Autodesk Inventor part; units mm, degrees
ref_plane "YZ Plane" through (0, 0, 0) normal (1, 0, 0) x (0, 1, 0)
ref_plane "XZ Plane" through (0, 0, 0) normal (0, 1, 0) x (-1, 0, 0)
ref_plane "XY Plane" through (0, 0, 0) normal (0, 0, 1) x (1, 0, 0)
sketch "Sketch1" plane through (0, 0, 0) normal (0, 0, 1) x (1, 0, 0)
  line L0 (-15.1742, 2.0557) -> (9.8258, 2.0557)
  line L1 (9.8258, 2.0557) -> (9.8258, -7.9443)
  line L2 (9.8258, -7.9443) -> (-15.1742, -7.9443)
  line L3 (-15.1742, -7.9443) -> (-15.1742, 2.0557)
  point P0 (0, 0)
  dimension "d0" = 25
  dimension "d1" = 10
extrude "Extrusion1" add sketch "Sketch1" along normal blind 5
sketch "Sketch2" plane through (0, 0, 5) normal (0, 0, 1) x (1, 0, 0)
  circle A0 centre (-10.1742, -2.9443) radius 1
  line L0 (-15.1742, 2.0557) -> (-15.1742, -7.9443)
  line L1 (9.8258, 2.0557) -> (-15.1742, 2.0557)
  line L2 (-2.6742, 2.0557) -> (-2.6742, -2.9443)
  circle A1 centre (4.8258, -2.9443) radius 1
  point P0 (0, 0)
  dimension "d4" = 2
  dimension "d5" = 5
  dimension "d6" = 5
hole "Hole1" at (-10.1742, -2.9443, 5) at (4.8258, -2.9443, 5) direction (0, 0, -1) diameter 2 end through all countersink diameter 6 countersink angle 90
sketch "Sketch3" plane through (0, 0, 5) normal (0, 0, 1) x (1, 0, 0)
  line L0 (9.8258, 2.0557) -> (-15.1742, 2.0557)
  line L1 (-15.1742, -7.9443) -> (9.8258, -7.9443)
  line L2 (-5.1742, 2.0557) -> (-0.1742, 2.0557)
  line L3 (-0.1742, 2.0557) -> (-0.1742, -7.9443)
  line L4 (-0.1742, -7.9443) -> (-5.1742, -7.9443)
  line L5 (-5.1742, -7.9443) -> (-5.1742, 2.0557)
  line L6 (-15.1742, 2.0557) -> (-15.1742, -7.9443)
  line L7 (9.8258, -7.9443) -> (9.8258, 2.0557)
  point P0 (0, 0)
  dimension "d14" = 10
  dimension "d15" = 10
extrude "Extrusion2" cut sketch "Sketch3" against normal blind 2 contours L3 L1 L5 L0
properties part number "CameraArmMount"
Source: CAD feature listing. Evaluate the final solid. Frame: model axes, mm. A direction names the side the tool comes from. Give positions to 0.01 mm unless a question says otherwise; leave off trailing zeros. Order: outer loops, then holes, each group sorted by start corner. A loop starts at its lowest first (then second) coordinate and runs counter-clockwise, first axis right, second up. Notation, with made-up numbers: (42, 55) -> (54, 55) arc R9 cw to (54, 69) -> close; hole circle Ø7 at (-36, 24.25). An arc over 180 degrees is marked (long way). Use a Markdown table: item, result.
Q1. First-contact query: P1, Ø4, axis at x = -3, y = -2, coming from the +Z side; P2, Ø2.5, axis at x = 4.83, y = -2.94, coming from the +Z side. Flat tips, straight axial feed; report the tip coordinate or a pass-through.
A:
| item | result |
|---|---|
| P1 | z = 3 |
| P2 | z = 3.26 |
Q2. Material intervals for line 1 (X direction, y = 1, z = 4.2); line 2 (X direction, y = -2.5, z = 3.1); line 3 (X direction, y = -1, z = 4.5), sorted ascending. Write a range as [from, to].
A:
| item | result |
|---|---|
| line 1 | [-15.17, -5.17], [-0.17, 9.83] |
| line 2 | [-15.17, -11.18], [-9.17, -5.17], [-0.17, 3.82], [5.83, 9.83] |
| line 3 | [-15.17, -11.75], [-8.6, -5.17], [-0.17, 3.25], [6.4, 9.83] |
Q3. Pull-direction query (Y, two-part tool) for faces 1 (the face through (-3, 2.056, 2)), 2 (the face through (-9.059, -2.798, 3.125)), 3 (the face through (5.71, -3.41, 1.48)), 4 (the face through (-3, -3, 0)); classes: +Y half, -Y half, draft (parallel to the pull), parting line (faces both ways), or undercut.
A:
| item | result |
|---|---|
| face 1 | +Y half |
| face 2 | undercut |
| face 3 | undercut |
| face 4 | draft |
Q4. Access query for faces 5 (the face through (-5.174, -3, 4)), 6 (the face through (-2, -7.944, 2)). Directions: +Z, -Z, +X, -X, +Y, -Y. A direction counts if a zero-diameter tool reaches every point of the face in a straight line with its end or side. Return the directions, or none.
A:
| item | result |
|---|---|
| face 5 | +Z, +Y, -Y |
| face 6 | +Z, -Z, +X, -X, -Y |
Q5. Section B-B (y = -7). Return the cut outline in (x, z), and give its area (3 significant figures).
A:
| item | result |
|---|---|
| outline | (-15.17, 0) -> (9.83, 0) -> (9.83, 5) -> (-0.17, 5) -> (-0.17, 3) -> (-5.17, 3) -> (-5.17, 5) -> (-15.17, 5) -> close |
| area | 115 mm^2 |
Q6. Section C-C (x = -1.5). Return the cut outline in (y, z), and give its area (3 significant figures).
A:
| item | result |
|---|---|
| outline | (-7.94, 0) -> (2.06, 0) -> (2.06, 3) -> (-7.94, 3) -> close |
| area | 30.0 mm^2 |
Q7. Section D-D (z = 2.2). Return the cut outline in (x, y), and give its area (3 significant figures).
A:
| item | result |
|---|---|
| outline | (-15.17, -7.94) -> (9.83, -7.94) -> (9.83, 2.06) -> (-15.17, 2.06) -> close; hole circle Ø2 at (-10.17, -2.94); hole circle Ø2 at (4.83, -2.94) |
| area | 244 mm^2 |
Q8. Section A-A (z = 4). Return the cut outline in (x, y).
A:
| item | result |
|---|---|
| outline | (-15.17, -7.94) -> (-5.17, -7.94) -> (-5.17, 2.06) -> (-15.17, 2.06) -> close; (-0.17, -7.94) -> (9.83, -7.94) -> (9.83, 2.06) -> (-0.17, 2.06) -> close; hole circle Ø4 at (-10.17, -2.94); hole circle Ø4 at (4.83, -2.94) |
